Geometry: final body of the model. Coordinates: model frame, mm. A direction names the side the tool comes from. Round coordinates to 2 decimals unless told otherwise and drop trailing zeros. Write each loop counter-clockwise with the first axis right and the second up, starting at its lowest first coordinate (ties: lowest second). Pieces come first, ordered by that corner, then holes. Notation, with made-up numbers: M -14.5,-28.75 L 7.5,-28.75 A7 ccw 7.5,-16.75 Z; hole C -35,-19 d7. An arc over 180 degrees is marked long. Use one line per item in the form item = value. Start each with the question number.
Item 1: Reachability of faces 1 (the flat face through (-5.474, 9.392, 3.219)), 2 (the flat face through (1, 9.4, 4.4)) from +Z, -Z, +X, -X, +Y, -Y: full face, straight path, thin tool, end or side. Return the list, or none.
Item 2: Section query D-D (z = -4.25). Return loops of the section in (x, y).
Item 3: Ray query, probe 1 along Z at (x, y) = (0, 14.75); probe 2 along X at (y, z) = (16, -1); probe 3 along Z at (x, y) = (-3, 16.5). Return the intervals inside material, ascending.
Item 4: Pull-direction query (Z, two-part tool) for faces 3 (the flat face through (-5.525, 9.392, -3.131)), 4 (the flat face through (-1, 9.4, 4.4)), 5 (the flat face through (0, 9, 6.35)); classes: pulls with the +Z half, pulls with the -Z half, needs draft (parallel to the pull), parting line crosses it, or undercut.
Item 5: Pin query (flat end, axial travel): pin 1 Ø1.5 at (y, z) = (11.5, -3.5) entering from +X; pin 2 Ø1.5 at (x, y) = (-4.5, 13) entering from -Z; pin 3 Ø1.5 at (y, z) = (6, 1) entering from +X. Return the tip coordinate at first contact, or that it passes through.
Item 6: Section query B-B (y = 1.75). Return loops of the section in (x, z), and give its area (3 significant figures).
Item 7: Section query A-A (x = 0). Return loops of the section in (y, z), and give its area (3 significant figures).
Item 8: Section query C-C (z = 0.5). Return loops of the section in (x, y), and give its area (3 significant figures).
Autodesk Inventor part; units mm, degrees
ref_plane "YZ Plane" through (0, 0, 0) normal (1, 0, 0) x (0, 1, 0)
ref_plane "XZ Plane" through (0, 0, 0) normal (0, 1, 0) x (-1, 0, 0)
ref_plane "XY Plane" through (0, 0, 0) normal (0, 0, 1) x (1, 0, 0)
sketch "Sketch1" plane through (0, 0, 0) normal (0, 1, 0) x (-1, 0, 0)
  line L0 (3.6662, 6.35) -> (7.3323, 0)
  line L1 (7.3323, 0) -> (3.6662, -6.35)
  line L2 (3.6662, -6.35) -> (-3.6662, -6.35)
  line L3 (-3.6662, -6.35) -> (-7.3323, 0)
  line L4 (-7.3323, 0) -> (-3.6662, 6.35)
  line L5 (-3.6662, 6.35) -> (3.6662, 6.35)
  arc A0 (-1, 3.873) -> (1, 3.873) centre (0, 0) ccw
  line L6 (1, 5) -> (-1, 5)
  line L7 (-1, 5) -> (-1, 3.873)
  line L8 (1, 5) -> (1, 3.873)
  dimension "d0" = 12.7
  dimension "d1" = 8
  dimension "d2" = 2
  dimension "d3" = 1
  dimension "d4" = 5
extrude "Extrusion1" add sketch "Sketch1" along normal blind 19.05
properties part number "500 Hex CIM adapter"
Working result:
q1.face_1 = +Z, -X, +Y, -Y
q1.face_2 = +Y, -Y
q2.outline = M -4.88,0 L 4.88,0 L 4.88,19.05 L -4.88,19.05 Z
q3.probe_1 = -6.35 to -4, 5 to 6.35
q3.probe_2 = -6.75 to -3.87, 3.87 to 6.75
q3.probe_3 = -6.35 to -2.65, 2.65 to 6.35
q4.face_3 = pulls with the -Z half
q4.face_4 = undercut
q4.face_5 = pulls with the +Z half
q5.pin_1 = 5.74
q5.pin_2 = -6.2
q5.pin_3 = 7.19
q6.outline = M -7.33,0 L -3.67,-6.35 L 3.67,-6.35 L 7.33,0 L 3.67,6.35 L -3.67,6.35 Z; hole M -1,3.87 A4 ccw long 1,3.87 L 1,5 L -1,5 Z
q6.area = 87.3 mm²
q7.outline = M 0,-6.35 L 19.05,-6.35 L 19.05,-4 L 0,-4 Z; M 0,5 L 19.05,5 L 19.05,6.35 L 0,6.35 Z
q7.area = 70.5 mm²
q8.outline = M -7.04,0 L -3.97,0 L -3.97,19.05 L -7.04,19.05 Z; M 3.97,0 L 7.04,0 L 7.04,19.05 L 3.97,19.05 Z
q8.area = 117 mm²
